Autodesk Inventor part; units mm, degrees
ref_plane "YZ Plane" through (0, 0, 0) normal (1, 0, 0) x (0, 1, 0)
ref_plane "XZ Plane" through (0, 0, 0) normal (0, 1, 0) x (-1, 0, 0)
ref_plane "XY Plane" through (0, 0, 0) normal (0, 0, 1) x (1, 0, 0)
sketch "Sketch1" plane through (0, 0, 0) normal (0, 1, 0) x (-1, 0, 0)
  line L0 (-22.05, -28.75) -> (22.05, -28.75)
  line L1 (22.05, -28.75) -> (22.05, 28.75)
  line L2 (22.05, 28.75) -> (-22.05, 28.75)
  line L3 (-22.05, 28.75) -> (-22.05, -28.75)
  line L4 (-22.05, -28.75) -> (22.05, 28.75) construction
  line L5 (22.05, -28.75) -> (-22.05, 28.75) construction
  point P0 (0, 0)
  dimension "d0" = 57.5
  dimension "d1" = 44.1
extrude "Extrusion1" add sketch "Sketch1" along normal blind 1.5
sketch "Sketch4" plane through (0, 1.5, 0) normal (0, 1, 0) x (1, 0, 0)
  line L0 (22.6381, -25.9185) -> (13.7388, -25.9185)
  line L1 (13.7388, -25.9185) -> (13.7388, -21.956)
  line L2 (13.7388, -21.956) -> (22.6381, -21.956)
  line L3 (22.6381, -21.956) -> (22.6381, -25.9185)
  line L4 (11.4165, -21.956) -> (0.7633, -21.956)
  line L5 (0.7633, -21.956) -> (0.7633, -24.4569)
  line L6 (0.7633, -24.4569) -> (11.4165, -24.4569)
  line L7 (11.4165, -24.4569) -> (11.4165, -21.956)
  line L8 (-0.6658, -26.6006) -> (-6.707, -26.6006)
  line L9 (-6.707, -26.6006) -> (-6.707, -22.3783)
  line L10 (-6.707, -22.3783) -> (-0.6658, -22.3783)
  line L11 (-0.6658, -22.3783) -> (-0.6658, -26.6006)
  line L12 (-6.707, -24.392) -> (-14.5426, -24.392)
  line L13 (-14.5426, -24.392) -> (-14.5426, -21.0953)
  line L14 (-14.5426, -21.0953) -> (-6.707, -21.0953)
  line L15 (-6.707, -21.0953) -> (-6.707, -24.392)
  line L16 (-14.5426, -21.0953) -> (-11.8996, -21.0953)
  line L17 (-11.8996, -21.0953) -> (-11.8996, -19.5363)
  line L18 (-11.8996, -19.5363) -> (-14.5426, -19.5363)
  line L19 (-14.5426, -19.5363) -> (-14.5426, -21.0953)
  line L20 (-21.1238, -24.2621) -> (-17.4211, -24.2621)
  line L21 (-17.4211, -24.2621) -> (-17.4211, -21.956)
  line L22 (-17.4211, -21.956) -> (-21.1238, -21.956)
  line L23 (-21.1238, -21.956) -> (-21.1238, -24.2621)
  line L24 (5.6616, -20.7705) -> (1.894, -20.7705)
  line L25 (1.894, -20.7705) -> (1.894, -17.3277)
  line L26 (1.894, -17.3277) -> (5.6616, -17.3277)
  line L27 (5.6616, -17.3277) -> (5.6616, -20.7705)
  line L28 (-2.848, -19.9261) -> (-5.2515, -19.9261)
  line L29 (-5.2515, -19.9261) -> (-5.2515, -18.3346)
  line L30 (-5.2515, -18.3346) -> (-2.848, -18.3346)
  line L31 (-2.848, -18.3346) -> (-2.848, -19.9261)
  line L32 (-17.2689, -17.0029) -> (-14.5426, -17.0029)
  line L33 (-14.5426, -17.0029) -> (-14.5426, -13.4952)
  line L34 (-14.5426, -13.4952) -> (-17.2689, -13.4952)
  line L35 (-17.2689, -13.4952) -> (-17.2689, -17.0029)
  line L36 (15.925, -11.4814) -> (12.4173, -11.4814)
  line L37 (12.4173, -11.4814) -> (12.4173, -14.7294)
  line L38 (12.4173, -14.7294) -> (15.925, -14.7294)
  line L39 (15.925, -14.7294) -> (15.925, -11.4814)
  line L40 (-2.1335, 9.0455) -> (1.894, 9.0455)
  line L41 (1.894, 9.0455) -> (1.894, -8.9481)
  line L42 (1.894, -8.9481) -> (-2.1335, -8.9481)
  line L43 (-2.1335, -8.9481) -> (-2.1335, 9.0455)
  line L44 (4.5573, 3.3291) -> (1.6991, 3.3291)
  line L45 (1.6991, 3.3291) -> (1.6991, 0.6009)
  line L46 (1.6991, 0.6009) -> (4.5573, 0.6009)
  line L47 (4.5573, 0.6009) -> (4.5573, 3.3291)
  line L48 (-17.5287, 13.7631) -> (-14.1519, 13.7631)
  line L49 (-14.1519, 13.7631) -> (-14.1519, 10.4096)
  line L50 (-14.1519, 10.4096) -> (-17.5287, 10.4096)
  line L51 (-17.5287, 10.4096) -> (-17.5287, 13.7631)
  line L52 (16.8052, 16.3739) -> (14.7212, 16.3739)
  line L53 (14.7212, 16.3739) -> (14.7212, 12.9633)
  line L54 (14.7212, 12.9633) -> (16.8052, 12.9633)
  line L55 (16.8052, 12.9633) -> (16.8052, 16.3739)
  line L56 (-23.3919, 26.0219) -> (-13.2211, 26.0219)
  line L57 (-13.2211, 26.0219) -> (-13.2211, 21.0711)
  line L58 (-13.2211, 21.0711) -> (-23.3919, 21.0711)
  line L59 (-23.3919, 21.0711) -> (-23.3919, 26.0219)
  line L60 (-20.3793, 16.7032) -> (-17.8455, 16.7032)
  line L61 (-17.8455, 16.7032) -> (-17.8455, 19.4346)
  line L62 (-17.8455, 19.4346) -> (-20.3793, 19.4346)
  line L63 (-20.3793, 19.4346) -> (-20.3793, 16.7032)
  line L64 (-11.1745, 21.8169) -> (-0.7032, 21.8169)
  line L65 (-0.7032, 21.8169) -> (-0.7032, 24.5446)
  line L66 (-0.7032, 24.5446) -> (-11.1745, 24.5446)
  line L67 (-11.1745, 24.5446) -> (-11.1745, 21.8169)
  line L68 (-2.5673, 18.6812) -> (-4.8458, 18.6812)
  line L69 (-4.8458, 18.6812) -> (-4.8458, 22.2038)
  line L70 (-4.8458, 22.2038) -> (-2.5673, 22.2038)
  line L71 (-2.5673, 22.2038) -> (-2.5673, 18.6812)
  line L72 (0.9146, 27.1153) -> (6.539, 27.1153)
  line L73 (6.539, 27.1153) -> (6.539, 22.2038)
  line L74 (6.539, 22.2038) -> (0.9146, 22.2038)
  line L75 (0.9146, 22.2038) -> (0.9146, 27.1153)
  line L76 (2.2307, 17.9158) -> (4.5573, 17.9158)
  line L77 (4.5573, 17.9158) -> (4.5573, 22.2038)
  line L78 (4.5573, 22.2038) -> (2.2307, 22.2038)
  line L79 (2.2307, 22.2038) -> (2.2307, 17.9158)
  line L80 (6.0899, 24.1958) -> (14.5454, 24.1958)
  line L81 (14.5454, 24.1958) -> (14.5454, 21.5323)
  line L82 (14.5454, 21.5323) -> (6.0899, 21.5323)
  line L83 (6.0899, 21.5323) -> (6.0899, 24.1958)
  line L84 (14.2886, 21.5323) -> (11.9019, 21.5323)
  line L85 (11.9019, 21.5323) -> (11.9019, 19.3557)
  line L86 (11.9019, 19.3557) -> (14.2886, 19.3557)
  line L87 (14.2886, 19.3557) -> (14.2886, 21.5323)
  line L88 (21.4363, 24.0758) -> (17.64, 24.0758)
  line L89 (17.64, 24.0758) -> (17.64, 21.5323)
  line L90 (17.64, 21.5323) -> (21.4363, 21.5323)
  line L91 (21.4363, 21.5323) -> (21.4363, 24.0758)
  point P0 (0, 0)
  point P1 (6.539, 24.1958)
  point P2 (6.0899, 22.2038)
extrude "Clearance Cutouts" [suppressed]
sketch "Sketch5" plane through (0, 1.5, 0) normal (0, 1, 0) x (1, 0, 0)
  line L0 (19.55, 25.75) -> (9.039, 25.75) construction
  line L1 (19.55, 26.75) -> (9.039, 26.75)
  line L2 (9.039, 24.75) -> (19.55, 24.75)
  arc A0 (19.55, 24.75) -> (19.55, 26.75) centre (19.55, 25.75) ccw
  arc A1 (9.039, 26.75) -> (9.039, 24.75) centre (9.039, 25.75) ccw
  line L3 (22.05, -28.75) -> (22.05, 28.75)
  line L4 (-2.5854, 25.75) -> (-10.7211, 25.75) construction
  line L5 (-2.5854, 24.75) -> (-10.7211, 24.75)
  line L6 (-10.7211, 26.75) -> (-2.5854, 26.75)
  arc A2 (-2.5854, 24.75) -> (-2.5854, 26.75) centre (-2.5854, 25.75) ccw
  arc A3 (-10.7211, 26.75) -> (-10.7211, 24.75) centre (-10.7211, 25.75) ccw
  line L7 (-19.55, -25.75) -> (-9.207, -25.75) construction
  line L8 (-22.05, -28.75) -> (22.05, -28.75)
  line L9 (-19.55, -26.75) -> (-9.207, -26.75)
  line L10 (-9.207, -24.75) -> (-19.55, -24.75)
  arc A4 (-19.55, -24.75) -> (-19.55, -26.75) centre (-19.55, -25.75) ccw
  arc A5 (-9.207, -26.75) -> (-9.207, -24.75) centre (-9.207, -25.75) ccw
  line L11 (-22.05, 28.75) -> (-22.05, -28.75)
  line L12 (2.8342, -25.75) -> (11.2388, -25.75) construction
  line L13 (2.8342, -26.75) -> (11.2388, -26.75)
  line L14 (11.2388, -24.75) -> (2.8342, -24.75)
  arc A6 (2.8342, -24.75) -> (2.8342, -26.75) centre (2.8342, -25.75) ccw
  arc A7 (11.2388, -26.75) -> (11.2388, -24.75) centre (11.2388, -25.75) ccw
  line L15 (22.05, 28.75) -> (-22.05, 28.75)
  point P0 (0, 0)
  point P1 (14.2945, 25.75)
  point P2 (8.039, 25.75)
  point P3 (20.55, 25.75)
  point P4 (-6.6533, 25.75)
  point P5 (-1.5854, 25.75)
  point P6 (-11.7211, 25.75)
  point P7 (-14.3785, -25.75)
  point P8 (-8.207, -25.75)
  point P9 (-20.55, -25.75)
  point P10 (7.0365, -25.75)
  point P11 (1.8342, -25.75)
  point P12 (12.2388, -25.75)
  dimension "d23" = 2
  dimension "d26" = 1.5
  dimension "d30" = 1
  dimension "d31" = 1
  dimension "d34" = 1.5
  dimension "d35" = 1
  dimension "d44" = 3
  dimension "d45" = 15.3967
  dimension "d46" = 10.1357
  dimension "d47" = 3
  dimension "d48" = 12.511
  dimension "d49" = 3
  dimension "d50" = 3
  dimension "d51" = 10.4046
  dimension "d52" = 9.8112
  dimension "d53" = 12.343
extrude "Extrusion4" cut sketch "Sketch5" against normal blind 1.5 contours A0 L2 A1 L1 | L5 A3 L6 A2 | A4 L10 A5 L9 | A6 L14 A7 L13
chamfer "Chamfer1" distance 2 angle 45 1 edges at (-22.05, 0.75, -28.75)
properties part number "Flex Holder V1 TPMockup" material "Thermoplastic Resin"
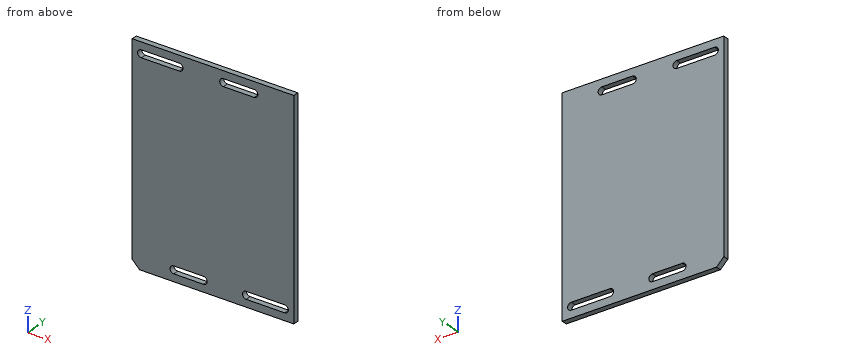
Work out the finished part from the listing and answer in its coordinate system (mm). Round coordinates to 2 decimals unless told otherwise and drop trailing zeros. Order: outer loops, then holes, each group sorted by start corner. A loop starts at its lowest first (then second) coordinate and runs counter-clockwise, first axis right, second up. Notation, with made-up numbers: M -30,17.25 L 25,17.25 A28 cw 25,39.25 Z; hole C 45.25,28.25 d3. An arc over 180 degrees is marked long. Put each result on its own line as item: value. Start each with the question number.
Q1. Section B-B, the plane z = -25.75 is taken. Write down the section's boundary in (x, y).
Q2. Section C-C, the plane x = -5 is taken. Write down the section's boundary in (y, z).
Q3. Section A-A, the plane y = 0.3 is taken. Write down the section's boundary in (x, z).
Q4. Straight lines are drawn through the part: L1, parallel to Z at x = 9.5, y = 0.8; L2, parallel to Z at x = 7, y = 0.75; L3, parallel to Z at x = -8.5, y = 1.2. For each, find the intervals that lie inside material, in ascending order. Write a range as [from, to].
Q5. Section D-D, the plane z = 25.75 is taken. Write down the section's boundary in (x, y), and give its area (3 significant figures).
Findings below:
1. outline: M -22.05,0 L -11.72,0 L -11.72,1.5 L -22.05,1.5 Z; M -1.59,0 L 8.04,0 L 8.04,1.5 L -1.59,1.5 Z; M 20.55,0 L 22.05,0 L 22.05,1.5 L 20.55,1.5 Z
2. outline: M 0,-28.75 L 1.5,-28.75 L 1.5,-26.75 L 0,-26.75 Z; M 0,-24.75 L 1.5,-24.75 L 1.5,28.75 L 0,28.75 Z
3. outline: M -22.05,-26.75 L -20.05,-28.75 L 22.05,-28.75 L 22.05,28.75 L -22.05,28.75 Z; hole M -19.55,24.75 L -9.21,24.75 A1 ccw -9.21,26.75 L -19.55,26.75 A1 ccw Z; hole M -10.72,-26.75 L -2.59,-26.75 A1 ccw -2.59,-24.75 L -10.72,-24.75 A1 ccw Z; hole M 2.83,24.75 L 11.24,24.75 A1 ccw 11.24,26.75 L 2.83,26.75 A1 ccw Z; hole M 9.04,-26.75 L 19.55,-26.75 A1 ccw 19.55,-24.75 L 9.04,-24.75 A1 ccw Z
4. L1: z = [-28.75, -26.75], [-24.75, 24.75], [26.75, 28.75]
4. L2: z = [-28.75, 24.75], [26.75, 28.75]
4. L3: z = [-28.75, -26.75], [-24.75, 25.04], [26.46, 28.75]
5. outline: M -22.05,0 L -20.55,0 L -20.55,1.5 L -22.05,1.5 Z; M -8.21,0 L 1.83,0 L 1.83,1.5 L -8.21,1.5 Z; M 12.24,0 L 22.05,0 L 22.05,1.5 L 12.24,1.5 Z
5. area: 32.0 mm^2
